from build123d import *

# Parameters (mm, degrees)
SKETCH1_R           = 8.3
BOSS_EXTRUDE1_DEPTH = 20
BOSS_EXTRUDE2_DEPTH = 25
SKETCH3_R           = 7
BOSS_EXTRUDE3_DEPTH = 20
SKETCH4_R           = 22.5
BOSS_EXTRUDE4_DEPTH = 10
SKETCH5_R           = 6
BOSS_EXTRUDE5_DEPTH = 28


with BuildPart() as part:
    # Sketch1 → Boss-Extrude1 (new body)
    with BuildSketch(Plane(origin=(0, 0, 0), x_dir=(1, 0, 0), z_dir=(0, 1, 0))):
        with Locations(Location((0, 0, 0), (0, 0, 270))):
            Circle(SKETCH1_R)
    extrude(amount=-BOSS_EXTRUDE1_DEPTH)

    # Sketch2 → Boss-Extrude2 (add)
    with BuildSketch(Plane(origin=(0, 0, 0), x_dir=(1, 0, 0), z_dir=(0, 1, 0))):
        Polygon((0, 13.856406461), (-12, 6.92820323), (-12, -6.92820323), (0, -13.856406461), (12, -6.92820323), (12, 6.92820323), align=None)
    extrude(amount=BOSS_EXTRUDE2_DEPTH)

    # Sketch3 → Boss-Extrude3 (add)
    with BuildSketch(Plane(origin=(0, 25, 0), x_dir=(1, 0, 0), z_dir=(0, 1, 0))):
        with Locations(Location((0, 0, 0), (0, 0, 270))):
            Circle(SKETCH3_R)
    extrude(amount=BOSS_EXTRUDE3_DEPTH)

    # Sketch4 → Boss-Extrude4 (add)
    with BuildSketch(Plane(origin=(0, 45, 0), x_dir=(1, 0, 0), z_dir=(0, 1, 0))):
        with Locations(Location((0, 0, 0), (0, 0, 270))):
            Circle(SKETCH4_R)
    extrude(amount=BOSS_EXTRUDE4_DEPTH)

    # Sketch5 → Boss-Extrude5 (add)
    with BuildSketch(Plane(origin=(0, 0, 0), x_dir=(0, 0, -1), z_dir=(1, 0, 0))):
        with Locations(Location((0, 12.5, 0), (0, 0, 180))):
            Circle(SKETCH5_R)
    extrude(amount=BOSS_EXTRUDE5_DEPTH)


solid = part.part
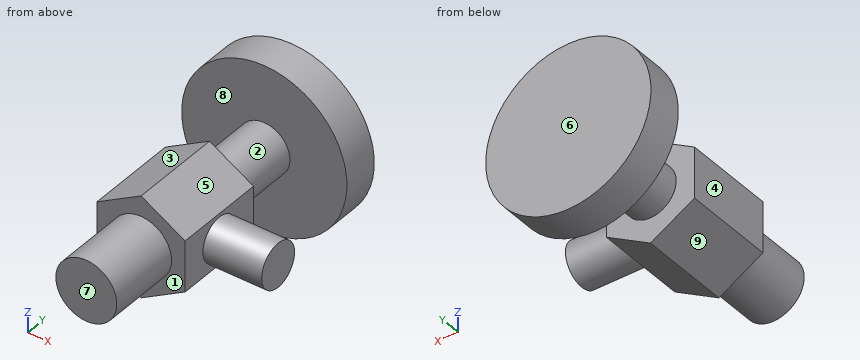
The model under review builds one solid part; all positions refer to its coordinate system, in mm. Face numbers are marked on the shaded views. A direction names the side the tool comes from. Give positions to 0.01 mm unless a question says otherwise; leave off trailing zeros. Write each loop counter-clockwise with the first axis right and the second up, starting at its lowest first coordinate (ties: lowest second). Pieces come first, ordered by that corner, then holes.
1. Add section A-A, the plane z = 0. Write out the cut boundary in (x, y), plus the area to 3 significant figures.
2. For P1, Ø1.5, axis at y = 39.5, z = -8.5, coming from the +X side; P2, Ø2, axis at x = 9, z = -17, coming from the -Y side; P3, Ø5, axis at y = 46, z = 2, coming from the +X side; P4, Ø12, axis at x = -17, y = 18.5, coming from the -Z side, all flat-tipped, find the tip position at first contact; note any pin that passes through.
3. Add section C-C, the plane z = -13. Write out the cut boundary in (x, y), plus the area to 3 significant figures.
4. Add section B-B, the plane y = 12.5. Write out the cut boundary in (x, z), plus the area to 3 significant figures.
5. Draft analysis for pull direction Y (two halves, no side actions). For the marked faces 6, 7, 8 and 9, state which applies: +Y half, -Y half, draft (parallel to the pull), parting line (faces both ways), or undercut.
6. Add section D-D, the plane x = 18.5. Write out the cut boundary in (y, z), plus the area to 3 significant figures.
7. Tool access review of the marked faces 1, 2, 3, 4 and 5: name each direction out of +Z, -Z, +X, -X, +Y, -Y from which nothing blocks a thin tool from reaching the whole face with its end or side.
8. Wall thickness on L1, parallel to Y at x = -11, z = -2; L2, parallel to Y at x = -6.5, z = 4; L3, parallel to X at y = 14, z = -2.5: over which ranges is each line inside the solid? List them lowest first.
Worked answers:
1. outline: (-22.5, 45) - (-7, 45) - (-7, 25) - (-12, 25) - (-12, 0) - (-8.3, 0) - (-8.3, -20) - (8.3, -20) - (8.3, 0) - (12, 0) - (12, 6.5) - (28, 6.5) - (28, 18.5) - (12, 18.5) - (12, 25) - (7, 25) - (7, 45) - (22.5, 45) - (22.5, 55) - (-22.5, 55) - close
1. area: 1,850 mm2
2. P1: passes through
2. P2: stops at y = 45
2. P3: stops at x = 22.5
2. P4: stops at z = -7.51
3. outline: (-18.36, 45) - (18.36, 45) - (18.36, 55) - (-18.36, 55) - close; (-1.48, 0) - (1.48, 0) - (1.48, 25) - (-1.48, 25) - close
3. area: 441 mm2
4. outline: (-12, -6.93) - (0, -13.86) - (12, -6.93) - (12, -6) - (28, -6) - (28, 6) - (12, 6) - (12, 6.93) - (0, 13.86) - (-12, 6.93) - close
4. area: 691 mm2
5. face 6: +Y half
5. face 7: -Y half
5. face 8: undercut
5. face 9: draft
6. outline: circle Ø12 at (12.5, 0); (45, -12.81) - (55, -12.81) - (55, 12.81) - (45, 12.81) - close
6. area: 369 mm2
7. face 1: -Y
7. face 2: none
7. face 3: +Z, -X, -Y
7. face 4: +Z, -Z, -X, -Y
7. face 5: +Z, +X, -Y
8. L1: y = 0 to 25, 45 to 55
8. L2: y = -20 to 25, 45 to 55
8. L3: x = -12 to 28
